Verification items for this drawing (mm, ordinates from the low corner). Round coordinates to 2 decimals unless told otherwise and drop trailing zeros. Order: outer loops, then holes, each group sorted by start corner. A loop starts at its lowest first (then second) coordinate and runs counter-clockwise, first axis right, second up. Notation, with made-up numbers: (-7, 78) -> (7, 78) arc R12 cw to (7, 92) -> close; hole circle Ø5 at (41, 22). An arc over 180 degrees is marked (long way). Answer in a Markdown table with one row per item. Add a question column.
1. Draft check along Y on the marked faces 1, 2 and 3. Enter one of: +Y half, -Y half, draft (parallel to the pull), parting line (faces both ways), or undercut.
2. Sectioned sample at A-A, the plane y = 6. Record the boundary of the cut face in (x, z) (3 decimals).
3. Material ranges on L1, parallel to X at y = 4.75, z = 25; L2, parallel to Y at x = 116.01, z = 26 (3 decimals); L3, parallel to X at y = 4.5, z = 12.5, recorded low to high. Write a range as from..to.
4. Depth check by flat-ended pin: P1, Ø4, axis at x = 116.01, y = 4.765, coming from the +Z side. Enter the tip coordinate at first touch or a pass-through.
5. Sectioned sample at C-C, the plane x = 27. Record the boundary of the cut face in (y, z) (3 decimals), then the cut area to 3 significant figures.
6. Sectioned sample at B-B, the plane x = 45. Record the boundary of the cut face in (y, z) (3 decimals).
7. Sectioned sample at D-D, the plane z = 2.5. Record the boundary of the cut face in (x, y) (3 decimals).
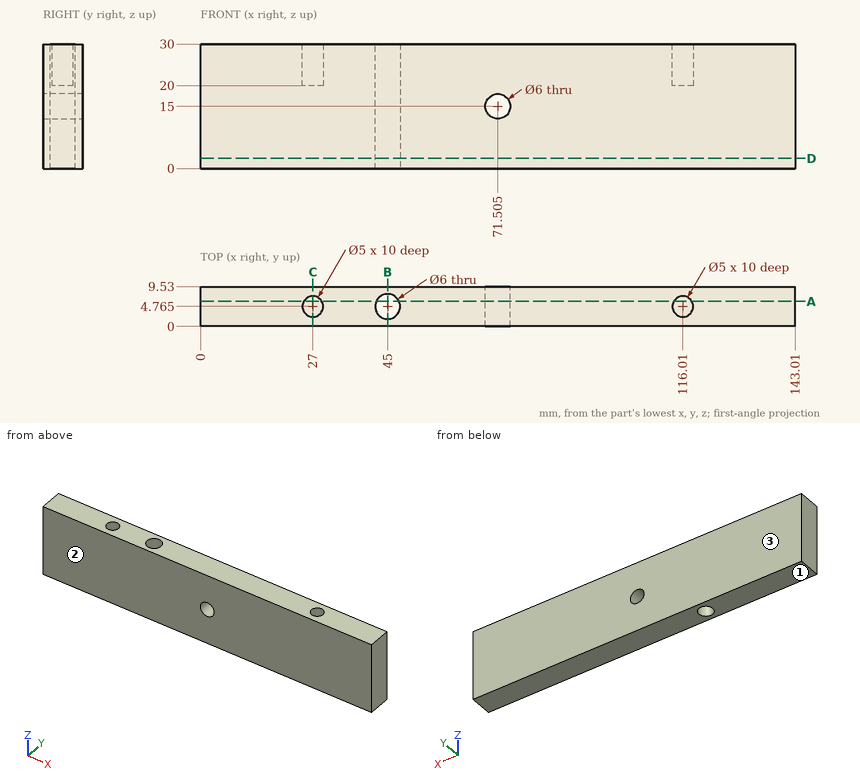
Answer key:
| question | item | result |
|---|---|---|
| 1 | face 1 | draft |
| 1 | face 2 | -Y half |
| 1 | face 3 | +Y half |
| 2 | outline | (0, 0) -> (42.266, 0) -> (42.266, 30) -> (29.174, 30) -> (29.174, 20) -> (24.826, 20) -> (24.826, 30) -> (0, 30) -> close; (47.734, 0) -> (143.01, 0) -> (143.01, 30) -> (118.184, 30) -> (118.184, 20) -> (113.836, 20) -> (113.836, 30) -> (47.734, 30) -> close; hole circle Ø6 at (71.505, 15) |
| 3 | L1 | x = 0..24.5, 29.5..42, 48..113.51, 118.51..143.01 |
| 3 | L2 | y = 0..2.265, 7.265..9.53 |
| 3 | L3 | x = 0..42.01, 47.99..69.85, 73.16..143.01 |
| 4 | P1 | stops at z = 20 |
| 5 | outline | (0, 0) -> (9.53, 0) -> (9.53, 30) -> (7.265, 30) -> (7.265, 20) -> (2.265, 20) -> (2.265, 30) -> (0, 30) -> close |
| 5 | area | 236 mm² |
| 6 | outline | (0, 0) -> (1.765, 0) -> (1.765, 30) -> (0, 30) -> close; (7.765, 0) -> (9.53, 0) -> (9.53, 30) -> (7.765, 30) -> close |
| 7 | outline | (0, 0) -> (143.01, 0) -> (143.01, 9.53) -> (0, 9.53) -> close; hole circle Ø6 at (45, 4.765) |
